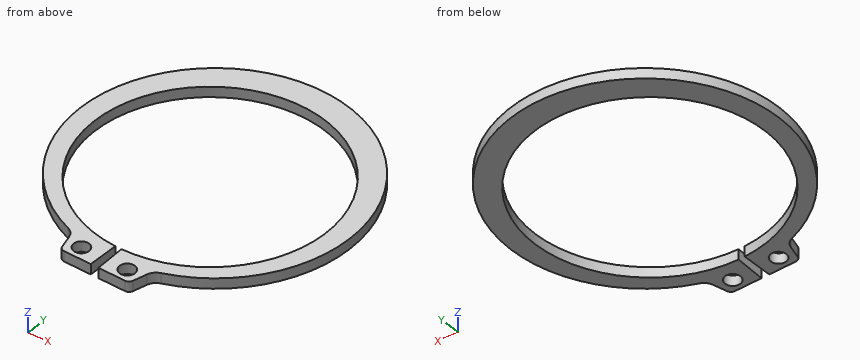
from build123d import *

# Parameters (mm, degrees)
SKETCH1_R           = 0.8001
BOSS_EXTRUDE1_DEPTH = 1.0668


with BuildPart() as part:
    # Sketch1 → Boss-Extrude1 (new body)
    with BuildSketch(Plane.XY):
        with BuildLine():
            Line((3.16619789, -15.718395078), (0.399594472, -15.718395078))
            Line((0.399594472, -15.718395078), (0.3175, -12.619595078))
            ThreePointArc((0.3175, -12.619595078), (0, 11.3538), (-0.3175, -12.619595078))
            Line((-0.3175, -12.619595078), (-0.399594472, -15.718395078))
            Line((-0.399594472, -15.718395078), (-3.16619789, -15.718395078))
            ThreePointArc((-3.16619789, -15.718395078), (-3.475448696, -15.613418575), (-3.65688821, -15.341875153))
            Line((-3.65688821, -15.341875153), (-4.02209585, -13.978901683))
            ThreePointArc((-4.02209585, -13.978901683), (-4.311388241, -13.450794656), (-4.811419846, -13.115301715))
            ThreePointArc((-4.811419846, -13.115301715), (0, 13.97), (4.811419846, -13.115301715))
            ThreePointArc((4.811419846, -13.115301715), (4.311388241, -13.450794656), (4.02209585, -13.978901683))
            Line((4.02209585, -13.978901683), (3.65688821, -15.341875153))
            ThreePointArc((3.65688821, -15.341875153), (3.475448696, -15.613418575), (3.16619789, -15.718395078))
        make_face()
        with Locations((-2.3749, -14.448395078)):
            Circle(SKETCH1_R, mode=Mode.SUBTRACT)
        with Locations((2.3749, -14.448395078)):
            Circle(SKETCH1_R, mode=Mode.SUBTRACT)
    extrude(amount=BOSS_EXTRUDE1_DEPTH)


solid = part.part
Check sheet for the modelled part. Datum: model origin and axes. Units: mm. Give positions to 0.01 mm unless a question says otherwise; leave off trailing zeros. Write each loop counter-clockwise with the first axis right and the second up, starting at its lowest first coordinate (ties: lowest second). Pieces come first, ordered by that corner, then holes. Notation, with made-up numbers: (37.5, 68) -> (89.5, 68) arc R30 cw to (89.5, 106) -> close; hole circle Ø2 at (-29.5, -2.75). An arc over 180 degrees is marked (long way). One line per item, written item: value. Start each with the question number.
Item 1: Section check A-A on x = 2.25. Record the cut outline in (y, z).
Item 2: Section check B-B on y = 5. Record the cut outline in (x, z), then the cut area to 3 significant figures.
Item 3: Section check D-D on z = 0.85. Record the cut outline in (x, y) (1 decimal).
Item 4: Material ranges on probe 1 along Y at (x, z) = (-3.5, 0.85); probe 2 along X at (y, z) = (-10.25, 0.95); probe 3 along Y at (x, z) = (9.25, 1), recorded low to high. Write a range as from..to.
Item 5: Section check C-C on x = 8. Record the cut outline in (y, z), then the cut area to 3 significant figures.
Results list:
1. outline: (-15.72, 0) -> (-15.24, 0) -> (-15.24, 1.07) -> (-15.72, 1.07) -> close; (-13.66, 0) -> (-12.41, 0) -> (-12.41, 1.07) -> (-13.66, 1.07) -> close; (11.14, 0) -> (13.79, 0) -> (13.79, 1.07) -> (11.14, 1.07) -> close
2. outline: (-13.04, 0) -> (-10.58, 0) -> (-10.58, 1.07) -> (-13.04, 1.07) -> close; (10.58, 0) -> (13.04, 0) -> (13.04, 1.07) -> (10.58, 1.07) -> close
2. area: 5.25 mm²
3. outline: (-4.8, -13.1) arc R1.3 cw to (-4, -14) -> (-3.7, -15.3) arc R0.5 ccw to (-3.2, -15.7) -> (-0.4, -15.7) -> (-0.3, -12.6) arc R12 cw (long way) to (0.3, -12.6) -> (0.4, -15.7) -> (3.2, -15.7) arc R0.5 ccw to (3.7, -15.3) -> (4, -14) arc R1.3 cw to (4.8, -13.1) arc R14 ccw (long way) to start; hole circle Ø1.6 at (-2.4, -14.4); hole circle Ø1.6 at (2.4, -14.4)
4. probe 1: -15.59..-12.1, 10.83..13.52
4. probe 2: -9.49..-7.16, 7.16..9.49
4. probe 3: -10.47..-8.26, 6.99..10.47
5. outline: (-11.45, 0) -> (-9.56, 0) -> (-9.56, 1.07) -> (-11.45, 1.07) -> close; (8.29, 0) -> (11.45, 0) -> (11.45, 1.07) -> (8.29, 1.07) -> close
5. area: 5.38 mm²
